CAD build for the part. Positions are in the model's coordinates, mm. A direction names the side the tool comes from. Round coordinates to 2 decimals unless told otherwise and drop trailing zeros. Write each loop counter-clockwise with the first axis right and the second up, starting at its lowest first coordinate (ties: lowest second). Pieces come first, ordered by that corner, then holes. Notation, with made-up numbers: (88, 23.25) - (128, 23.25) arc R32 ccw to (128, 59.25) - close; hole circle Ø9 at (-4, 62.5). An arc over 180 degrees is marked (long way). Answer in a Markdown table with one row per item.
Autodesk Inventor part; units mm, degrees
ref_plane "YZ Plane" through (0, 0, 0) normal (1, 0, 0) x (0, 1, 0)
ref_plane "XZ Plane" through (0, 0, 0) normal (0, 1, 0) x (-1, 0, 0)
ref_plane "XY Plane" through (0, 0, 0) normal (0, 0, 1) x (1, 0, 0)
sketch "Sketch1" plane through (0, 0, 0) normal (0, 0, 1) x (1, 0, 0)
  line L0 (0, 0) -> (1219.2, 0)
  line L1 (1181.1, 0) -> (1181.1, 609.6)
  line L2 (1181.1, 1219.2) -> (0, 0)
  line L3 (0, 0) -> (590.55, 609.6)
  line L4 (590.55, 520.7) -> (590.55, 481.8325)
  line L5 (590.55, 481.8325) -> (123.7747, 0)
  line L6 (590.55, 609.6) -> (1181.1, 609.6)
  line L7 (1181.1, 520.7) -> (590.55, 520.7)
  dimension "d0" = 88.9
  dimension "d1" = 88.9
extrude "Extrusion1" add sketch "Sketch1" against normal blind 38.1 contours L2 L6 L1 L7 L4 L5 L0
properties part number "side-side1"
Q1. Saw through at A-A on z = -6. List the corners of the cut face in (x, y), then the cut area to 3 significant figures.
Computed:
| item | result |
|---|---|
| outline | (0, 0) - (123.77, 0) - (590.55, 481.83) - (590.55, 520.7) - (1181.1, 520.7) - (1181.1, 609.6) - (590.55, 609.6) - close |
| area | 120,000 mm2 |
Q2. Saw through at B-B on x = 894.5. List the corners of the cut face in (y, z).
Computed:
| item | result |
|---|---|
| outline | (520.7, -38.1) - (609.6, -38.1) - (609.6, 0) - (520.7, 0) - close |
Q3. Flat gauge pins, fed straight in: pin 1 (10 mm diameter, centred on x = 570.5, z = -11.5, fed in from +Y); pin 2 (11.5 mm diameter, centred on x = 896.5, z = -12, fed in from -Y); pin 3 (19 mm diameter, centred on y = 502, z = -15, fed in from +X). Where does each tip first touch, or does it go through?
Computed:
| item | result |
|---|---|
| pin 1 | stops at y = 594.06 |
| pin 2 | stops at y = 520.7 |
| pin 3 | stops at x = 590.55 |
Q4. Drill centre lines: line 1 (Y direction, x = 698, z = -4); line 2 (Y direction, x = 247, z = -33.5); line 3 (X direction, y = 107.5, z = -13.5). Where is each one in solid material? Low to high.
Computed:
| item | result |
|---|---|
| line 1 | y = 520.7 to 609.6 |
| line 2 | y = 127.2 to 254.97 |
| line 3 | x = 104.14 to 227.92 |
Q5. 3-axis set-ups, long thin cutter, end or side, ignore diameter. For faces 1 (the flat face through (544, 442, -38.1)), 2 (the flat face through (590.55, 502, -19)): which of +Z, -Z, +X, -X, +Y, -Y reach the whole face in a straight line?
Computed:
| item | result |
|---|---|
| face 1 | -Z, +X, -X, +Y, -Y |
| face 2 | +Z, -Z, +X, -Y |
Q6. Saw through at C-C on y = 401. List the corners of the cut face in (x, z).
Computed:
| item | result |
|---|---|
| outline | (388.47, -38.1) - (512.24, -38.1) - (512.24, 0) - (388.47, 0) - close |
